Could you check a few things on this drawing? It's one solid part, dimensions in mm from its lowest x, y, z. Round coordinates to 2 decimals unless told otherwise and drop trailing zeros. Write each loop counter-clockwise with the first axis right and the second up, starting at its lowest first coordinate (ties: lowest second). Pieces come first, ordered by that corner, then holes. Notation, with made-up numbers: (88, 49.25) -> (144, 49.25) arc R16 cw to (144, 71.25) -> close; hole circle Ø4 at (65.25, 24). An arc over 180 degrees is marked (long way). Put each result on its own line as item: value. Start each with the question number.
1) If I drill on line 1 along Z through (x, y) = (136, 6.9); line 2 along X through (y, z) = (6.85, 2.5); line 3 along Y through (x, z) = (9, 58.5), over which ranges is the centre line in solid material (lowest first)? Write a range as [from, to].
2) I want a section at A-A, the plane x = 136. List the corners of the cut face in (y, z) for me.
3) I want a section at B-B, the plane z = 51. List the corners of the cut face in (x, y) for me.
4) Will these pins go through, and if not, where does the flat tip stop? P1, Ø2, axis at x = 112, y = 5.5, coming from the -Z side; P2, Ø3.5, axis at x = 2.5, z = 98, coming from the -Y side; P3, Ø1.3, axis at y = 8.5, z = 63.5, coming from the +X side; P4, Ø3, axis at x = 121, y = 4, coming from the +Z side.
5) I want a section at D-D, the plane x = 54. List the corners of the cut face in (y, z) for me.
6) I want a section at C-C, the plane y = 2.5. List the corners of the cut face in (x, z) for me, then the cut area to 3 significant figures.
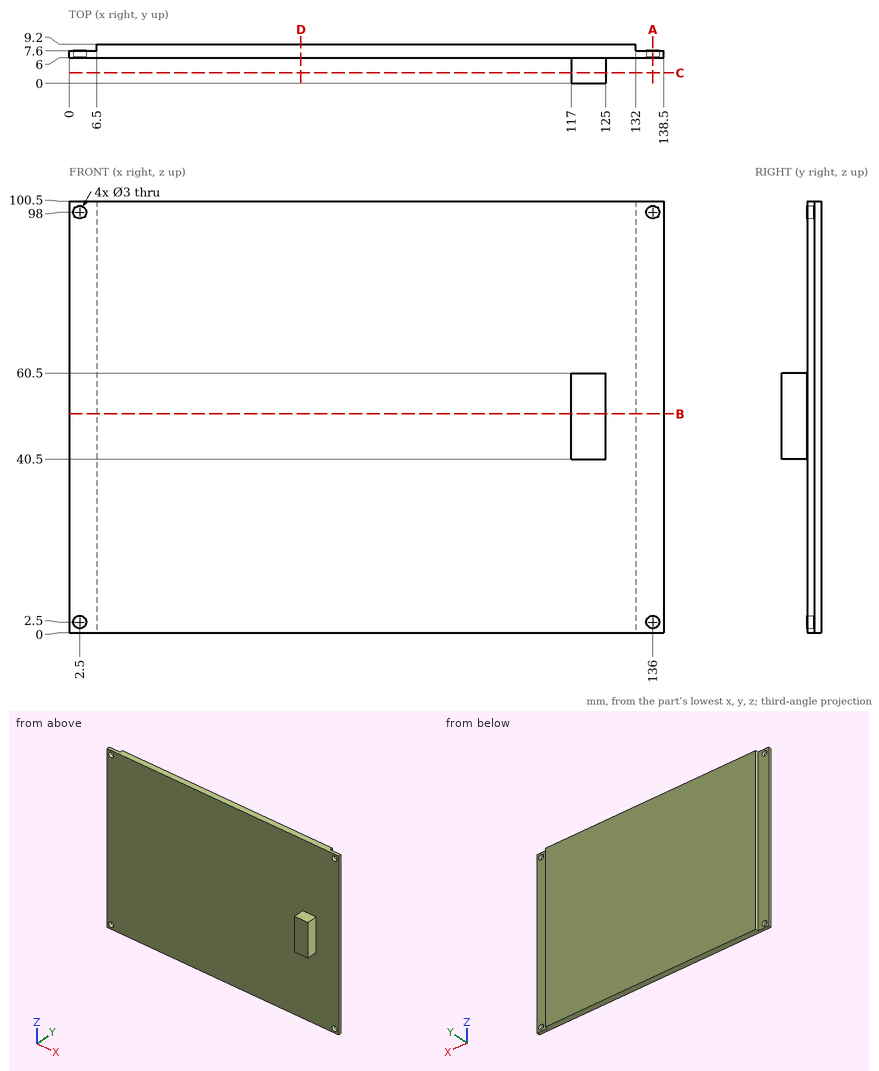
Findings:
1. line 1: z = [0, 1], [4, 96.5], [99.5, 100.5]
1. line 2: x = [0, 1], [4, 134.5], [137.5, 138.5]
1. line 3: y = [6, 9.2]
2. outline: (6, 0) -> (7.6, 0) -> (7.6, 1) -> (6, 1) -> close; (6, 4) -> (7.6, 4) -> (7.6, 96.5) -> (6, 96.5) -> close; (6, 99.5) -> (7.6, 99.5) -> (7.6, 100.5) -> (6, 100.5) -> close
3. outline: (0, 6) -> (117, 6) -> (117, 0) -> (125, 0) -> (125, 6) -> (138.5, 6) -> (138.5, 7.6) -> (132, 7.6) -> (132, 9.2) -> (6.5, 9.2) -> (6.5, 7.6) -> (0, 7.6) -> close
4. P1: stops at z = 0
4. P2: stops at y = 6
4. P3: stops at x = 132
4. P4: stops at z = 60.5
5. outline: (6, 0) -> (9.2, 0) -> (9.2, 100.5) -> (6, 100.5) -> close
6. outline: (117, 40.5) -> (125, 40.5) -> (125, 60.5) -> (117, 60.5) -> close
6. area: 160 mm2
